The listing builds one solid part. Answer for the finished solid, in the listing's coordinates (mm). Round coordinates to 2 decimals unless told otherwise and drop trailing zeros. Loops run counter-clockwise (first coordinate to the right, second up) from the corner with the lowest first, then second, coordinate; pieces in that order, holes last. Notation, with made-up numbers: (46.5, -39) - (96.5, -39) arc R30 cw to (96.5, 0) - close; hole circle Ø9 at (38, 6.25). An arc over 180 degrees is marked (long way). One line per item, written item: value.
```python
from build123d import *

# Parameters (mm, degrees)
F0_R     = 6
F1_DEPTH = 101
F2_R     = 5
F4_START = -55
F3_W     = 4.994883243
F3_H     = 25
F3_W_2   = 5.9151866052
F3_W_3   = 8.303230216
F4_DEPTH = 453


# Not quite as in the source:
# - a feature names something its author has since deleted; it is built from what else it names


with BuildPart() as f1:
    # F0 (on Top) → F1 (new body)
    with BuildSketch(Plane.XY):
        with BuildLine():
            Line((254.0328107559, 6.2914491919), (-253.9614388373, 8.7085508081))
            Line((-253.9614388373, 8.7085508081), (-254.1422456511, -29.2910190433))
            Line((-254.1422456511, -29.2910190433), (-8.0838477514, -19.3235865814))
            ThreePointArc((-8.0838477514, -19.3235865814), (-0.4142050626, -11.0063405813), (7.9030409375, -18.67598327))
            Line((7.9030409375, -18.67598327), (253.9614388373, -8.7085508081))
            Line((253.9614388373, -8.7085508081), (254.0328107559, 6.2914491919))
        make_face()
        with Locations((-241.9818616233, -11.1859360032)):
            Circle(F0_R, mode=Mode.SUBTRACT)
        with BuildLine():
            ThreePointArc((7.9030409375, -18.67598327), (-0.4142050626, -11.0063405813), (-8.0838477514, -19.3235865814))
            Line((-8.0838477514, -19.3235865814), (-5.0863061222, -19.2021609605))
            ThreePointArc((-5.0863061222, -19.2021609605), (-0.2927794417, -14.0038822105), (4.9054993084, -18.7974088909))
            Line((4.9054993084, -18.7974088909), (7.9030409375, -18.67598327))
        make_face()
        with BuildLine():
            Line((-5.0863061222, -19.2021609605), (-8.0838477514, -19.3235865814))
            ThreePointArc((-8.0838477514, -19.3235865814), (0.0715305988, -26.9981458439), (7.9095965931, -18.9997849257))
            ThreePointArc((7.9095965931, -18.9997849257), (7.9079575113, -18.83785092), (7.9030409375, -18.67598327))
            Line((7.9030409375, -18.67598327), (4.9054993084, -18.7974088909))
            ThreePointArc((4.9054993084, -18.7974088909), (4.908572167, -18.8985761721), (4.9095965931, -18.9997849257))
            ThreePointArc((4.9095965931, -18.9997849257), (0.0108053467, -23.9987604996), (-5.0863061222, -19.2021609605))
        make_face()
    extrude(amount=F1_DEPTH)

    # F2
    f2_edges = [f1.edges().sort_by_distance(p)[0] for p in [
        (-254.142246, -29.291019, 50.5),
        (-253.961439, 8.708551, 50.5),
    ]]
    fillet(f2_edges, radius=F2_R)

    # F3 (on face) → F4 (cut)
    with BuildSketch(Plane(origin=(-253.9971247966, 1.2085508081, 0), x_dir=(-0.004758074, -0.9999886803, 0), z_dir=(-0.9999886803, 0.004758074, 0)).offset(F4_START)):
        with Locations((27.7658584427, 52.5)):
            Rectangle(F3_W, F3_H)
        with Locations((22.3108235186, 52.5)):
            Rectangle(F3_W_2, F3_H)
        with Locations((15.201615108, 52.5)):
            Rectangle(F3_W_3, F3_H)
    extrude(amount=-F4_DEPTH, mode=Mode.SUBTRACT)


solid = f1.part
```
1) Each of these flat-tipped pins is pushed along its axis until it touches: pin 1 Ø2 at (x, z) = (-89, 65.5) entering from +Y; pin 2 Ø3 at (y, z) = (-17, 53) entering from -X; pin 3 Ø1.5 at (y, z) = (3, 89.5) entering from -X; pin 4 Ø7 at (x, y) = (-241.98, -11.19) entering from -Z. Where does it stop, or does it pass through?
Final values:
pin 1: y = 7.93
pin 2: x = -254.09
pin 3: x = -253.99
pin 4: through
2) For a pull along Y with two mould halves and no side action, classify faces 1 (the cylindrical face through (-246.74, -14.84, 49.79)), 2 (the flat face through (-130.19, -24.27, 38.57)), 3 (the flat face through (-98, -15, 65)) as released by +Y, released by -Y, zero draft, split by the parting line, or undercut.
Final values:
face 1: undercut
face 2: released by -Y
face 3: zero draft
3) A cutting plane is placed at B-B on z = 31. Give the vertices of the cut face in (x, y), and give its area (3 significant figures).
Final values:
outline: (-254.12, -24.06) arc R5 ccw to (-248.92, -29.08) - (-8.08, -19.32) arc R8 ccw to (7.9, -18.68) - (253.96, -8.71) - (254.03, 6.29) - (-248.96, 8.68) arc R5 ccw to (-253.99, 3.71) - close; hole circle Ø12 at (-241.98, -11.19); hole circle Ø10 at (-0.09, -19)
area: 13,400 mm2
4) A cutting plane is placed at A-A on x = 47. Give the vertices of the cut face in (y, z).
Final values:
outline: (-17.09, 0) - (7.28, 0) - (7.28, 101) - (-17.09, 101) - (-17.09, 65) - (-11.27, 65) - (-11.27, 40) - (-17.09, 40) - close
5) A cutting plane is placed at C-C on x = 146. Give the vertices of the cut face in (y, z), and give its area (3 significant figures).
Final values:
outline: (-13.08, 0) - (6.81, 0) - (6.81, 101) - (-13.08, 101) - (-13.08, 65) - (-11.74, 65) - (-11.74, 40) - (-13.08, 40) - close
area: 1,980 mm2
6) Consider L1, parallel to Y at x = -4.5, z = 21; L2, parallel to X at y = 0, z = 90; L3, parallel to Y at x = -77, z = 77. Determine where each line is inside the solid, lowest interval first.
Final values:
L1: -25.67 to -21.36, -16.64 to 7.52
L2: -254 to 254
L3: -22.12 to 7.87
